Check sheet for the modelled part. Datum: model origin and axes. Units: mm. Give positions to 0.01 mm unless a question says otherwise; leave off trailing zeros. Put each result on its own line as item: value. Start each with the question number.
```python
from build123d import *

# Parameters (mm, degrees)
SKETCH1_W           = 185
SKETCH1_H           = 116
BOSS_EXTRUDE1_DEPTH = 3
SKETCH8_R           = 1.5
CUT_EXTRUDE3_DEPTH  = 3
SKETCH10_R          = 1.2
SKETCH10_R_2        = 1.1
SKETCH10_R_3        = 2.5
SKETCH10_R_4        = 5
SKETCH10_R_5        = 12.80026957
CUT_EXTRUDE6_DEPTH  = 3
SKETCH11_W          = 10
SKETCH11_H          = 3
CUT_EXTRUDE7_DEPTH  = 3
SKETCH13_R          = 1.5
SKETCH13_R_2        = 1.506866353
CUT_EXTRUDE8_DEPTH  = 3


with BuildPart() as part:
    # Sketch1 → Boss-Extrude1 (new body)
    with BuildSketch(Plane(origin=(0, 0, 0), x_dir=(1, 0, 0), z_dir=(0, 1, 0))):
        Rectangle(SKETCH1_W, SKETCH1_H)
    extrude(amount=BOSS_EXTRUDE1_DEPTH)

    # Sketch8 → Cut-Extrude3 (cut)
    with BuildSketch(Plane(origin=(0, 3, 0), x_dir=(1, 0, 0), z_dir=(0, 1, 0))):
        with Locations(Location((-62.764720309, 18.264176016, 0), (0, 0, 270))):
            Circle(SKETCH8_R)
        with Locations(Location((-63.016694441, -21.735030339, 0), (0, 0, 270))):
            Circle(SKETCH8_R)
        with Locations(Location((7.284285639, 25.823062556, 0), (0, 0, 270))):
            Circle(SKETCH8_R)
        with Locations(Location((6.931521854, -30.175826341, 0), (0, 0, 270))):
            Circle(SKETCH8_R)
    extrude(amount=-CUT_EXTRUDE3_DEPTH, mode=Mode.SUBTRACT)

    # Sketch10 → Cut-Extrude6 (cut)
    with BuildSketch(Plane(origin=(0, 3, 0), x_dir=(1, 0, 0), z_dir=(0, 1, 0))):
        with Locations(Location((52.862616564, 8.568904476, 0), (0, 0, 270))):
            Circle(SKETCH10_R)
        with Locations(Location((52.862616564, -13.331095524, 0), (0, 0, 270))):
            Circle(SKETCH10_R_2)
        with Locations(Location((76.362616564, -13.331095524, 0), (0, 0, 270))):
            Circle(SKETCH10_R_2)
        with Locations(Location((76.362616564, 8.568904476, 0), (0, 0, 270))):
            Circle(SKETCH10_R_2)
        with Locations(Location((55.812578484, 27.817001132, 0), (0, 0, 270))):
            Circle(SKETCH10_R_3)
        with Locations(Location((72.735814959, 27.817001132, 0), (0, 0, 270))):
            Circle(SKETCH10_R_4)
        with Locations(Location((30, -9.5, 0), (0, 0, 270))):
            Circle(SKETCH10_R_5)
        with BuildLine():
            Line((50.912616564, -8.231095524), (53.912616564, -8.231095524))
            ThreePointArc((53.912616564, -8.231095524), (54.619723345, -8.523988743), (54.912616564, -9.231095524))
            Line((54.912616564, -9.231095524), (54.912616564, -16.581095524))
            Line((54.912616564, -16.581095524), (74.312616564, -16.581095524))
            Line((74.312616564, -16.581095524), (74.312616564, -9.381095524))
            ThreePointArc((74.312616564, -9.381095524), (74.605509783, -8.673988743), (75.312616564, -8.381095524))
            Line((75.312616564, -8.381095524), (77.712616564, -8.381095524))
            Line((77.712616564, -8.381095524), (77.712616564, 3.618904476))
            Line((77.712616564, 3.618904476), (75.312616564, 3.618904476))
            ThreePointArc((75.312616564, 3.618904476), (74.605509783, 3.911797695), (74.312616564, 4.618904476))
            Line((74.312616564, 4.618904476), (74.312616564, 11.818904476))
            Line((74.312616564, 11.818904476), (54.912616564, 11.818904476))
            Line((54.912616564, 11.818904476), (54.912616564, 4.473317322))
            ThreePointArc((54.912616564, 4.473317322), (54.620243085, 3.766730663), (53.914087151, 3.473318403))
            Line((53.914087151, 3.473318403), (50.912616564, 3.468904476))
            Line((50.912616564, 3.468904476), (50.912616564, -8.231095524))
        make_face()
    extrude(amount=-CUT_EXTRUDE6_DEPTH, mode=Mode.SUBTRACT)

    # Sketch11 → Cut-Extrude7 (cut)
    with BuildSketch(Plane(origin=(0, 3, 0), x_dir=(1, 0, 0), z_dir=(0, 1, 0))):
        with Locations((-47.5, 54.5)):
            Rectangle(SKETCH11_W, SKETCH11_H)
        with Locations((42.5, 54.5)):
            Rectangle(SKETCH11_W, SKETCH11_H)
        with Locations((-47.5, -54.5)):
            Rectangle(SKETCH11_W, SKETCH11_H)
        with Locations((42.5, -54.5)):
            Rectangle(SKETCH11_W, SKETCH11_H)
    extrude(amount=-CUT_EXTRUDE7_DEPTH, mode=Mode.SUBTRACT)

    # Sketch13 → Cut-Extrude8 (cut)
    with BuildSketch(Plane.XZ):
        with Locations(Location((56, -54.5, 0), (0, 0, 270))):
            Circle(SKETCH13_R)
        with Locations(Location((-60.935816723, -54.506866353, 0), (0, 0, 270))):
            Circle(SKETCH13_R_2)
        with Locations(Location((-61, 54.5, 0), (0, 0, 270))):
            Circle(SKETCH13_R)
        with Locations(Location((56, 54.5, 0), (0, 0, 270))):
            Circle(SKETCH13_R)
    extrude(amount=-CUT_EXTRUDE8_DEPTH, mode=Mode.SUBTRACT)


solid = part.part
```
Q1. Section check A-A, the plane y = 0.6. Give the number of separate pieces and of enclosed holes in the cut face, then the cut area to 3 significant figures.
Q2. Mould release check, pull along X, two halves, no side actions. Record for faces 1 (the face through (-1, 3, -1)), 2 (the face through (33.84, 1.52, 21.71)): pulls with the +X half, pulls with the -X half, needs draft (parallel to the pull), parting line crosses it, or undercut.
Q3. Thickness scan on line 1 along X through (y, z) = (0.75, -54.5); line 2 along Z through (x, y) = (46, 2.3); line 3 along X through (y, z) = (1.8, -5). Record the ranges inside material, lowest first. Write a range as [from, to].
Found:
1. separate pieces: 1
1. enclosed holes: 20
1. area: 20,000 mm^2
2. face 1: needs draft
2. face 2: undercut
3. line 1: x = [-92.5, -62.44], [-59.43, -52.5], [-42.5, 37.5], [47.5, 54.5], [57.5, 92.5]
3. line 2: z = [-58, -56], [-53, 53], [56, 58]
3. line 3: x = [-92.5, 54.91], [74.31, 92.5]
